from build123d import *

# Parameters (mm, degrees)
F0_R     = 10
F1_DEPTH = 6.35
F2_W     = 124.221875
F2_H     = 111.91875
F2_R     = 10
F3_DEPTH = 6.351


# Not quite as in the source:
# - a feature names something its author has since deleted; it is built from what else it names


with BuildPart() as f1:
    # F0 (on Top) → F1 (new body)
    with BuildSketch(Plane.XY):
        Polygon((50.8, -55.959375), (50.8, 55.959375), (-50.8, 55.959375), (-152.4, 55.959375), (-152.4, -55.959375), (-50.8, -55.959375), align=None)
        with Locations((-101.6, 0)):
            Circle(F0_R, mode=Mode.SUBTRACT)
        Circle(F0_R, mode=Mode.SUBTRACT)
    extrude(amount=F1_DEPTH)

    # F2 (on face) → F3 (cut, through all)
    with BuildSketch(Plane.XY.offset(6.35)):
        with Locations((-11.3109375, 0)):
            Rectangle(F2_W, F2_H)
        Circle(F2_R, mode=Mode.SUBTRACT)
    extrude(amount=-F3_DEPTH, mode=Mode.SUBTRACT)


solid = f1.part
Part model, mm, in its own coordinate system. Coordinates: 2 decimals unless noted, no trailing zeros. Order: outer loops, then holes, each group sorted by start corner. A loop starts at its lowest first (then second) coordinate and runs counter-clockwise, first axis right, second up.
(1) Slice it at B-B, the plane x = -101.6. Write the cut outline in (y, z), and give its area (3 significant figures).
Check sheet entries:
outline: (-55.96, 0) - (-10, 0) - (-10, 6.35) - (-55.96, 6.35) - close; (10, 0) - (55.96, 0) - (55.96, 6.35) - (10, 6.35) - close
area: 584 mm2
(2) Slice it at A-A, the plane y = 0. Write the cut outline in (x, z), and give its area (3 significant figures).
Check sheet entries:
outline: (-152.4, 0) - (-111.6, 0) - (-111.6, 6.35) - (-152.4, 6.35) - close; (-91.6, 0) - (-73.42, 0) - (-73.42, 6.35) - (-91.6, 6.35) - close
area: 375 mm2
(3) Slice it at C-C, the plane z = 4.5. Write the cut outline in (x, y).
Check sheet entries:
outline: (-152.4, -55.96) - (-73.42, -55.96) - (-73.42, 55.96) - (-152.4, 55.96) - close; hole circle Ø20 at (-101.6, 0)
(4) Pull direction Y, two halves, no side cores. Call faces 1 (the face through (-112, 55.959, 3)), 2 (the face through (-92.363, -3.83, 3.131)), 3 (the face through (-113, 1, 0)): pulls with the +Y half, pulls with the -Y half, needs draft (parallel to the pull), parting line crosses it, or undercut.
Check sheet entries:
face 1: pulls with the +Y half
face 2: undercut
face 3: needs draft
(5) Probe L1, parallel to Y at x = -101.6, z = 2. List the from-to ranges inside material, lowest first.
Check sheet entries:
L1: y = -55.96 to -10, 10 to 55.96
